Here's how the part is built. I have some questions about the finished solid (model axes, mm). Coordinates: 2 decimals unless noted, no trailing zeros. Write each loop counter-clockwise with the first axis right and the second up, starting at its lowest first coordinate (ties: lowest second). Pieces come first, ordered by that corner, then holes.
Item 1: If we section it at A-A (x = -15.5): Please give me the cut outline in (y, z), then the cut area to 3 significant figures.
Item 2: If I drill on line 1 (Y direction, x = 32, z = 66.5); line 2 (Y direction, x = 21, z = 12), over which ranges is the centre line in solid material (lowest first)?
Item 3: I'm going to push flat-ended pins straight in: pin 1 Ø6 at (x, z) = (-38, 47.5) entering from -Y; pin 2 Ø16.5 at (y, z) = (-77.5, 8.5) entering from +X; pin 3 Ø1.6 at (y, z) = (-80, 1) entering from +X; pin 4 Ø1.6 at (y, z) = (-80, 1) entering from -X. Where does each tip first touch, or does it pass through?
Item 4: If we section it at B-B (z = 55): Please give me the cut outline in (x, y).
Item 5: If we section it at C-C (x = -55): Please give me the cut outline in (y, z), then the cut area to 3 significant figures.
from build123d import *

# Parameters (mm, degrees)
F1_DEPTH = 83
F2_DEPTH = 1.5
F0_W     = 130
F0_H     = 1.5
F3_DEPTH = 15


with BuildPart() as f1:
    # F0 (on Top) → F1 (new body)
    with BuildSketch(Plane.XY):
        Polygon((75, -70), (75, 70), (-75, 70), (-75, -70), (-65, -70), (65, -70), align=None)
    extrude(amount=F1_DEPTH)



with BuildPart() as f2:
    # F0 (on Top) → F2 (new body)
    with BuildSketch(Plane.XY):
        with BuildLine():
            Line((65, -85), (65, -71.5))
            Line((65, -71.5), (-65, -71.5))
            Line((-65, -71.5), (-65, -85))
            Line((-65, -85), (-57, -85))
            Line((-57, -85), (-57, -75))
            ThreePointArc((-57, -75), (-55, -73), (-53, -75))
            Line((-53, -75), (-53, -85))
            Line((-53, -85), (-44.5, -85))
            Line((-44.5, -85), (-44.5, -75))
            ThreePointArc((-44.5, -75), (-42.5, -73), (-40.5, -75))
            Line((-40.5, -75), (-40.5, -85))
            Line((-40.5, -85), (53, -85))
            Line((53, -85), (53, -75))
            ThreePointArc((53, -75), (55, -73), (57, -75))
            Line((57, -75), (57, -85))
            Line((57, -85), (65, -85))
        make_face()
    extrude(amount=F2_DEPTH)


with BuildPart() as f1_1:
    add(f1.part)

    add(f2.part)  # F3 merges F2
    # F0 (on Top) → F3 (join)
    with BuildSketch(Plane.XY):
        with Locations((0, -70.75)):
            Rectangle(F0_W, F0_H)
    extrude(amount=F3_DEPTH)


solid = f1_1.part
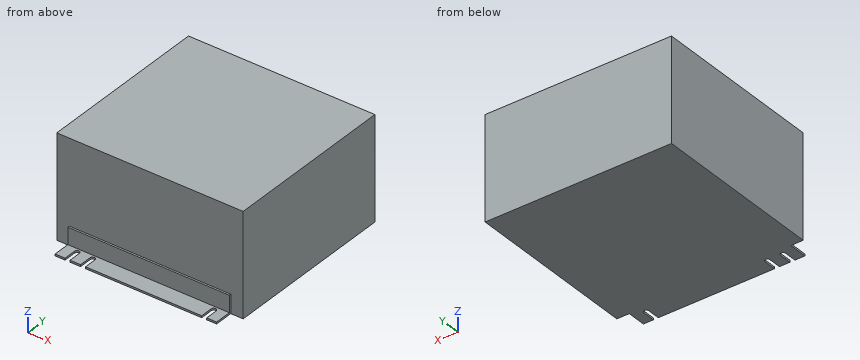
Answer list:
1. outline: (-85, 0) - (70, 0) - (70, 83) - (-70, 83) - (-70, 15) - (-71.5, 15) - (-71.5, 1.5) - (-85, 1.5) - close
1. area: 11,700 mm2
2. line 1: y = -70 to 70
2. line 2: y = -71.5 to 70
3. pin 1: stops at y = -70
3. pin 2: stops at x = 75
3. pin 3: stops at x = 65
3. pin 4: stops at x = -65
4. outline: (-75, -70) - (75, -70) - (75, 70) - (-75, 70) - close
5. outline: (-73, 0) - (70, 0) - (70, 83) - (-70, 83) - (-70, 15) - (-71.5, 15) - (-71.5, 1.5) - (-73, 1.5) - close
5. area: 11,600 mm2
